Part model, mm, in its own coordinate system. A direction names the side the tool comes from. Round coordinates to 2 decimals unless told otherwise and drop trailing zeros. Write each loop counter-clockwise with the first axis right and the second up, starting at its lowest first coordinate (ties: lowest second). Pieces come first, ordered by that corner, then holes. Notation, with made-up numbers: M -28.75,16.5 L -6.75,16.5 A23 cw -6.75,40.5 Z; hole C 14.25,33 d7. An arc over 180 degrees is marked long. Use a Markdown table: item, result. Add a question column.
1) Drop flat-ended pins along their axis: P1, Ø3, axis at x = 67.5, y = -6.5, coming from the -Z side; P2, Ø6, axis at x = 88.5, y = -31, coming from the +Z side; P3, Ø3, axis at y = -48, z = 58, coming from the +X side; P4, Ø5, axis at y = -50.5, z = 57, coming from the -X side. Give the stop position or say it passes through.
2) Slice it at C-C on x = 63.5. Write the cut outline in (y, z) (1 decimal).
3) Slice it at A-A on z = 41.5. Write the cut outline in (x, y), plus the area to 3 significant figures.
4) Wall check: probe 1 along Y at (x, z) = (55, 55.5); probe 2 along Z at (x, y) = (37, 8) (3 decimals); probe 3 along X at (y, z) = (-58.5, 40). Give the ranges that are in metal, low to high.
5) Slice it at B-B on x = 32.5. Write the cut outline in (y, z) (3 decimals).
6) Two-plate mould, pull along Z, no slides. Class faces 4 (the face through (144.1, -28, 0)), 5 (the face through (54, -50, 51.435)), 6 (the face through (99, 15, -7.62)): released by +Z, released by -Z, zero draft, split by the parting line, or undercut.
7) Slice it at D-D on x = 129. Write the cut outline in (y, z), plus the area to 3 significant figures.
8) Which spindle directions (+Z, -Z, +X, -X, +Y, -Y) get a long thin tool onto all of the face, cutting with end or side? Do faces 1 (the face through (129, -38.1, -5)), 2 (the face through (136, -19.429, 8)), 3 (the face through (141.288, -31, 8)). Say none if no direction does.
Autodesk Inventor part; units mm, degrees
ref_plane "YZ Plane" through (0, 0, 0) normal (1, 0, 0) x (0, 1, 0)
ref_plane "XZ Plane" through (0, 0, 0) normal (0, 1, 0) x (-1, 0, 0)
ref_plane "XY Plane" through (0, 0, 0) normal (0, 0, 1) x (1, 0, 0)
sketch "Sketch1" plane through (0, 0, 0) normal (0, 0, 1) x (1, 0, 0)
  line L0 (0, -53.3468) -> (0, -11.9835)
  line L1 (68.5887, -53.3468) -> (0, -53.3468)
  line L2 (68.5887, 0) -> (68.5887, -53.3468)
  line L3 (0, 0) -> (68.5887, 0)
  line L4 (0, -2.1686) -> (0, 0)
  line L5 (0, -11.9835) -> (0, -2.1686)
  circle A0 centre (15.2894, -50.7921) radius 1.5631
  circle A1 centre (14.0269, -2.6176) radius 1.4996
  line L6 (0, 0) -> (68.5887, 0)
  line L7 (68.5887, 0) -> (68.5887, -53.3468)
  line L8 (68.5887, -53.3468) -> (0, -53.3468)
  line L9 (0, -53.3468) -> (0, 0)
  circle A2 centre (14.0269, -2.6176) radius 1.4996
  circle A3 centre (15.2894, -50.7921) radius 1.5631
extrude "Extrusion1" add sketch "Sketch1" against normal blind 5.08 contours A0 | A1
ref_plane "Work Plane1" through (0, 0, 0) normal (0, 0, 1) x (1, 0, 0)
sketch "Sketch2" plane through (0, 0, 0) normal (0, 0, 1) x (1, 0, 0)
  line L0 (0, -53.3468) -> (0, -11.9835)
  line L1 (68.5887, 0) -> (68.5887, -53.3468)
  line L2 (0, -2.1686) -> (0, 0)
  line L3 (0, 0) -> (0, -53.3468)
  line L4 (68.5887, -53.3468) -> (68.5887, 0)
  line L5 (68.5887, -71.3254) -> (144.1005, -71.3254)
  line L6 (144.1005, -71.3254) -> (144.1005, 16.6007)
  line L7 (144.1005, 16.6007) -> (68.5887, 16.6007)
  line L8 (68.5887, 16.6007) -> (68.5887, -71.3254)
  line L9 (68.5887, 16.6007) -> (0, 16.6007)
  line L10 (0, 16.6007) -> (0, 0)
  line L11 (68.5887, -71.3254) -> (0, -71.3254)
  line L12 (0, -71.3254) -> (0, -53.3468)
extrude "Extrusion2" add sketch "Sketch2" along normal mid plane 5.08
sketch "Sketch3" plane through (0, 0, -2.54) normal (0, 0, -1) x (-1, 0, 0)
  line L0 (-125.7496, -4.4471) -> (-125.7496, -55.0115)
  line L1 (0, -71.3254) -> (-144.1005, -71.3254)
  line L2 (-125.7496, -38.1) -> (-133.2651, -38.1)
  line L3 (-133.2651, -38.1) -> (-133.2651, -17.4625)
  line L4 (-133.2651, -17.4625) -> (-125.7496, -17.4625)
  line L5 (-125.7496, -17.4625) -> (-125.7496, -38.1)
  line L6 (-125.7462, 13.1821) -> (-71.1251, 13.1821)
  line L7 (0, 16.6007) -> (-144.1005, 16.6007)
  line L8 (-92.075, 13.1821) -> (-104.775, 13.1821)
  line L9 (-104.775, 13.1821) -> (-104.775, 16.6007)
  line L10 (-104.775, 16.6007) -> (-92.075, 16.6007)
  line L11 (-92.075, 16.6007) -> (-92.075, 13.1821)
  line L12 (-80.6496, -69.3179) -> (-97.3996, -69.3179)
  line L13 (-144.1005, -71.3254) -> (0, -71.3254)
  line L14 (-97.3996, -69.3179) -> (-84.496, -69.3179)
  line L15 (-84.496, -69.3179) -> (-84.496, -71.3254)
  line L16 (-84.496, -71.3254) -> (-97.3996, -71.3254)
  line L17 (-97.3996, -71.3254) -> (-97.3996, -69.3179)
  point P0 (0, 0)
  point P1 (-68.5887, -71.3254)
  point P2 (-68.5887, 16.6007)
extrude "Extrusion3" add sketch "Sketch3" along normal blind 5.08
sketch "Sketch9" plane through (0, 0, 2.54) normal (0, 0, 1) x (1, 0, 0)
  line L0 (0, -71.3254) -> (7.9375, -71.3254)
  line L1 (7.9375, -71.3254) -> (7.9375, -52.2754)
  line L2 (7.9375, -52.2754) -> (0, -52.2754)
  line L3 (0, -52.2754) -> (0, -71.3254)
  line L4 (0, 16.6007) -> (7.9502, 16.6007)
  line L5 (7.9502, 16.6007) -> (7.9502, -2.4493)
  line L6 (7.9502, -2.4493) -> (0, -2.4493)
  line L7 (0, -2.4493) -> (0, 16.6007)
  line L8 (76.2, -71.3254) -> (84.1502, -71.3254)
  line L9 (84.1502, -71.3254) -> (84.1502, -52.2754)
  line L10 (84.1502, -52.2754) -> (76.2, -52.2754)
  line L11 (76.2, -52.2754) -> (76.2, -71.3254)
  line L12 (76.2, 16.6007) -> (84.1502, 16.6007)
  line L13 (84.1502, 16.6007) -> (84.1502, -2.4493)
  line L14 (84.1502, -2.4493) -> (76.2, -2.4493)
  line L15 (76.2, -2.4493) -> (76.2, 16.6007)
  line L16 (144.1005, 16.6007) -> (0, 16.6007)
  line L17 (0, -71.3254) -> (144.1005, -71.3254)
  point P0 (0, 0)
  dimension "d19" = 7.9502
  dimension "d20" = 19.05
  dimension "d21" = 7.9502
  dimension "d22" = 19.05
  dimension "d23" = 7.9502
  dimension "d24" = 19.05
  dimension "d41" = 19.05
extrude "Extrusion7" add sketch "Sketch9" along normal blind 67.945
sketch "Sketch10" plane through (0, 0, 2.54) normal (0, 0, 1) x (1, 0, 0)
  line L0 (141.2875, -13.0792) -> (131.7625, -13.0792)
  line L1 (131.7625, -13.0792) -> (131.7625, -19.4292)
  line L2 (131.7625, -19.4292) -> (141.2875, -19.4292)
  line L3 (141.2875, -19.4292) -> (141.2875, -13.0792)
  line L4 (141.2875, -22.6042) -> (131.7625, -22.6042)
  line L5 (131.7625, -22.6042) -> (131.7625, -25.7792)
  line L6 (131.7625, -25.7792) -> (141.2875, -25.7792)
  line L7 (141.2875, -25.7792) -> (141.2875, -22.6042)
  line L8 (141.2875, -28.9542) -> (131.7625, -28.9542)
  line L9 (131.7625, -28.9542) -> (131.7625, -32.1292)
  line L10 (131.7625, -32.1292) -> (141.2875, -32.1292)
  line L11 (141.2875, -32.1292) -> (141.2875, -28.9542)
  line L12 (144.1005, 16.6007) -> (84.1502, 16.6007)
  line L13 (84.1502, -71.3254) -> (144.1005, -71.3254)
  line L14 (90.4875, -27.3667) -> (109.5375, -27.3667)
  point P0 (0, 0)
  dimension "d30" = 3.175
  dimension "d31" = 3.175
  dimension "d32" = 3.175
  dimension "d33" = 3.175
  dimension "d39" = 6.35
  dimension "d70" = 43.9674
extrude "Extrusion8" add sketch "Sketch10" along normal blind 10.16
sketch "Sketch11" plane through (0, 0, 70.485) normal (0, 0, 1) x (1, 0, 0)
  line L0 (0, 16.6007) -> (84.1502, 16.6007)
  line L1 (84.1502, 16.6007) -> (84.1502, -2.4493)
  line L2 (84.1502, -2.4493) -> (0, -2.4493)
  line L3 (0, -2.4493) -> (0, 16.6007)
  line L4 (0, -71.3254) -> (7.9375, -71.3254)
  line L5 (0, -71.3254) -> (84.1502, -71.3254)
  line L6 (84.1502, -71.3254) -> (84.1502, -52.2754)
  line L7 (84.1502, -52.2754) -> (0, -52.2754)
  line L8 (0, -52.2754) -> (0, -71.3254)
  point P0 (0, 0)
  dimension "d44" = 19.05
  dimension "d45" = 19.05
extrude "Extrusion9" add sketch "Sketch11" along normal blind 9.525
sketch "Sketch12" plane through (0, 0, 70.485) normal (0, 0, -1) x (-1, 0, 0)
  line L0 (0, 16.6007) -> (-92.075, 16.6007)
  line L1 (-84.1375, 16.6007) -> (-39.6875, 16.6007)
  line L2 (-39.6875, 16.6007) -> (-39.6875, 20.6375)
  line L3 (-39.6875, 20.6375) -> (-84.1375, 20.6375)
  line L4 (-84.1375, 20.6375) -> (-84.1375, 16.6007)
  line L5 (-84.1375, -6.4861) -> (-39.6875, -6.4861)
  line L6 (-39.6875, -6.4861) -> (-39.6875, -2.4493)
  line L7 (-39.6875, -2.4493) -> (-84.1375, -2.4493)
  line L8 (-84.1375, -2.4493) -> (-84.1375, -6.4861)
  line L9 (-84.1375, -52.2754) -> (-39.6875, -52.2754)
  line L10 (-39.6875, -52.2754) -> (-39.6875, -48.2386)
  line L11 (-39.6875, -48.2386) -> (-84.1375, -48.2386)
  line L12 (-84.1375, -48.2386) -> (-84.1375, -52.2754)
  line L13 (-84.1375, -75.3622) -> (-39.6875, -75.3622)
  line L14 (-39.6875, -75.3622) -> (-39.6875, -71.3254)
  line L15 (-39.6875, -71.3254) -> (-84.1375, -71.3254)
  line L16 (-84.1375, -71.3254) -> (-84.1375, -75.3622)
  line L17 (0, -2.4493) -> (-84.1502, -2.4493)
  line L18 (-84.1502, -52.2754) -> (0, -52.2754)
  line L19 (0, -71.3254) -> (-84.1502, -71.3254)
  line L20 (0, -2.4493) -> (0, -52.2754)
  line L21 (-39.6875, -52.2754) -> (0, -52.2754)
  line L22 (0, -52.2754) -> (0, -45.9254)
  line L23 (0, -45.9254) -> (-39.6875, -45.9254)
  line L24 (-39.6875, -45.9254) -> (-39.6875, -52.2754)
  line L25 (-39.6875, -2.4493) -> (0, -2.4493)
  line L26 (0, -2.4493) -> (0, -8.7993)
  line L27 (0, -8.7993) -> (-39.6875, -8.7993)
  line L28 (-39.6875, -8.7993) -> (-39.6875, -2.4493)
  point P0 (0, 0)
  dimension "d46" = 4.0368
  dimension "d53" = 44.45
  dimension "d54" = 6.35
  dimension "d55" = 6.35
extrude "Extrusion10" add sketch "Sketch12" along normal blind 19.05 and the other way blind 9.525
sketch "Sketch13" plane through (0, -45.9254, 51.435) normal (0, 1, 0) x (1, 0, 0)
  line L0 (19.1249, 12.586) -> (19.1249, -9.639) construction
  line L1 (15.9499, 12.586) -> (15.9499, -9.639)
  line L2 (22.2999, -9.639) -> (22.2999, 12.586)
  arc A0 (22.2999, 12.586) -> (15.9499, 12.586) centre (19.1249, 12.586) ccw
  arc A1 (15.9499, -9.639) -> (22.2999, -9.639) centre (19.1249, -9.639) ccw
  point P0 (0, 51.435)
  point P1 (19.1249, 1.4735)
extrude "Extrusion11" cut sketch "Sketch13" against normal blind 8.255
sketch "Sketch14" plane through (0, -8.7993, 51.435) normal (0, -1, 0) x (1, 0, 0)
  line L0 (19.1249, 12.586) -> (19.1249, -9.639) construction
  line L1 (15.9499, 12.586) -> (15.9499, -9.639)
  line L2 (22.2999, -9.639) -> (22.2999, 12.586)
  arc A0 (22.2999, 12.586) -> (15.9499, 12.586) centre (19.1249, 12.586) ccw
  arc A1 (15.9499, -9.639) -> (22.2999, -9.639) centre (19.1249, -9.639) ccw
  point P0 (0, 51.435)
  point P1 (19.1249, 1.4735)
extrude "Extrusion12" cut sketch "Sketch14" against normal blind 8.255
sketch "Sketch15" plane through (39.6875, -6.4861, 51.435) normal (0, -1, 0) x (1, 0, 0)
  circle A0 centre (23.8125, 14.2875) radius 4.7625
  line L0 (-31.7373, -48.895) -> (-31.7373, 19.05)
  circle A1 centre (-31.7373, 14.2875) radius 4.7625
  point P0 (-39.6875, -51.435)
  dimension "d64" = 9.525
extrude "Extrusion13" add sketch "Sketch15" along normal blind 44.45
properties part number "RC_Chassis"
Entries:
| question | item | result |
|---|---|---|
| 1 | P1 | stops at z = -2.54 |
| 1 | P2 | stops at z = 2.54 |
| 1 | P3 | stops at x = 84.14 |
| 1 | P4 | stops at x = 0 |
| 2 | outline | M -75.4,51.4 L -71.3,51.4 L -71.3,70.5 L -52.3,70.5 L -52.3,51.4 L -48.2,51.4 L -48.2,61 L -6.5,61 L -6.5,51.4 L -2.4,51.4 L -2.4,70.5 L 16.6,70.5 L 16.6,51.4 L 20.6,51.4 L 20.6,80 L -6.5,80 L -6.5,70.5 L -48.2,70.5 L -48.2,80 L -75.4,80 Z; M -71.3,-2.5 L 16.6,-2.5 L 16.6,2.5 L -71.3,2.5 Z |
| 3 | outline | M 0,-71.33 L 7.94,-71.33 L 7.94,-52.28 L 0,-52.28 Z; M 0,-2.45 L 7.95,-2.45 L 7.95,16.6 L 0,16.6 Z; M 76.2,-71.33 L 84.15,-71.33 L 84.15,-52.28 L 76.2,-52.28 Z; M 76.2,-2.45 L 84.15,-2.45 L 84.15,16.6 L 76.2,16.6 Z |
| 3 | area | 606 mm^2 |
| 4 | probe 1 | y = -75.36 to -71.33, -52.28 to -48.24, -6.49 to -2.45, 16.6 to 20.64 |
| 4 | probe 2 | z = -2.54 to 2.54, 70.485 to 80.01 |
| 4 | probe 3 | x = 0 to 7.94, 76.2 to 84.15 |
| 5 | outline | M -71.325,-2.54 L 16.601,-2.54 L 16.601,2.54 L -71.325,2.54 Z; M -71.325,70.485 L -52.275,70.485 L -52.275,51.435 L -45.925,51.435 L -45.925,80.01 L -71.325,80.01 Z; M -8.799,51.435 L -2.449,51.435 L -2.449,70.485 L 16.601,70.485 L 16.601,80.01 L -8.799,80.01 Z |
| 6 | face 4 | zero draft |
| 6 | face 5 | undercut |
| 6 | face 6 | released by -Z |
| 7 | outline | M -71.33,-2.54 L -38.1,-2.54 L -38.1,-7.62 L -17.46,-7.62 L -17.46,-2.54 L 16.6,-2.54 L 16.6,2.54 L -71.33,2.54 Z |
| 7 | area | 552 mm^2 |
| 8 | face 1 | -Z, +X, -X, -Y |
| 8 | face 2 | +Z, +X, -X |
| 8 | face 3 | +Z, +X, +Y, -Y |
